```python
from build123d import *

# Parameters (mm, degrees)
BOSS_EXTRUDE1_DEPTH   = 2
BOSS_EXTRUDE2_DEPTH   = 8
SKETCH3_W             = 1.099637712
SKETCH3_H             = 0.808368405
BOSS_EXTRUDE3_DEPTH   = 6
SKETCH4_W             = 1.099637712
SKETCH4_H             = 0.808368405
BOSS_EXTRUDE4_DEPTH   = 6
SKETCH5_W             = 1.099637712
SKETCH5_H             = 0.808368405
BOSS_EXTRUDE5_DEPTH   = 6
SKETCH6_W             = 1.099637712
SKETCH6_H             = 0.808368405
BOSS_EXTRUDE6_DEPTH   = 6
SKETCH7_W             = 4.9
SKETCH7_H             = 6.4
BOSS_EXTRUDE7_DEPTH   = 5
F_1_CLEARANCE_HOLE1_D = 2.20000068
CHAMFER1_SIZE         = 0.2
CHAMFER2_SIZE         = 0.8
FILLET1_R             = 0.8


# Read off the part's stored shape, not the designer's step: Cut-Extrude1, Cut-Extrude2
with BuildPart() as part:
    # Sketch1 → Boss-Extrude1 (new body)
    with BuildSketch(Plane(origin=(0, 0, -2), x_dir=(-1, 0, 0), z_dir=(0, 0, -1))):
        with BuildLine():
            Line((-1.910632622, 9.092570703), (-9.810632622, 9.092570703))
            Line((-9.810632622, 9.092570703), (-9.810632622, 1.192570703))
            ThreePointArc((-9.810632622, 1.192570703), (-11.910632622, -0.907429297), (-9.810632622, -3.007429297))
            Line((-9.810632622, -3.007429297), (-9.810632622, -10.907429297))
            Line((-9.810632622, -10.907429297), (-1.910632622, -10.907429297))
            ThreePointArc((-1.910632622, -10.907429297), (0.189367378, -13.007429297), (2.289367378, -10.907429297))
            Line((2.289367378, -10.907429297), (10.189367378, -10.907429297))
            Line((10.189367378, -10.907429297), (10.189367378, -3.007429297))
            ThreePointArc((10.189367378, -3.007429297), (12.289367378, -0.907429297), (10.189367378, 1.192570703))
            Line((10.189367378, 1.192570703), (10.189367378, 9.092570703))
            Line((10.189367378, 9.092570703), (2.289367378, 9.092570703))
            ThreePointArc((2.289367378, 9.092570703), (0.189367378, 11.192570703), (-1.910632622, 9.092570703))
        make_face()
    extrude(amount=-BOSS_EXTRUDE1_DEPTH)

    # Sketch2 → Boss-Extrude2 (add)
    with BuildSketch(Plane.XY):
        Polygon((-2.670547611, -4.020890836), (-2.670547611, -6.129443348), (-8.453284272, -6.129443348), (-8.453284272, 4.602710154), (-2.670547611, 4.602710154), (-2.670547611, 2.494157643), (-3.670547611, 2.494157643), (-3.670547611, 3.602710154), (-7.453284272, 3.602710154), (-7.453284272, -5.129443348), (-3.670547611, -5.129443348), (-3.670547611, -4.020890836), align=None)
    extrude(amount=BOSS_EXTRUDE2_DEPTH)

    # Sketch3 → Boss-Extrude3 (add)
    with BuildSketch(Plane.XY):
        with Locations((-5.206678265, -1.71002656)):
            Rectangle(SKETCH3_W, SKETCH3_H)
    extrude(amount=BOSS_EXTRUDE3_DEPTH)

    # Sketch4 → Boss-Extrude4 (add)
    with BuildSketch(Plane.XY):
        with Locations((-5.206678265, 2.28997344)):
            Rectangle(SKETCH4_W, SKETCH4_H)
    extrude(amount=BOSS_EXTRUDE4_DEPTH)

    # Sketch5 → Boss-Extrude5 (add)
    with BuildSketch(Plane.XY):
        with Locations((-5.206678265, 0.289973441)):
            Rectangle(SKETCH5_W, SKETCH5_H)
    extrude(amount=BOSS_EXTRUDE5_DEPTH)

    # Sketch6 → Boss-Extrude6 (add)
    with BuildSketch(Plane.XY):
        with Locations((-5.206678265, -3.71002656)):
            Rectangle(SKETCH6_W, SKETCH6_H)
    extrude(amount=BOSS_EXTRUDE6_DEPTH)

    # Sketch7 → Boss-Extrude7 (add)
    with BuildSketch(Plane(origin=(0, 0, -2), x_dir=(-1, 0, 0), z_dir=(0, 0, -1))):
        with Locations((-5.779682622, -0.907429297)):
            Rectangle(SKETCH7_W, SKETCH7_H)
    extrude(amount=BOSS_EXTRUDE7_DEPTH)

    # Cut-Extrude1 outline → Cut-Extrude1 (revolve, cut)
    with BuildSketch(Plane(origin=(5.83567735, -2.101434569, 0), x_dir=(1, 0, 0), z_dir=(0, -1, 0))):
        with BuildLine():
            Line((0.75, -7), (0.75, -6))
            ThreePointArc((0.75, -6), (0.530330086, -6.530330086), (0, -6.75))
            Line((0, -6.75), (0, -7))
            Line((0, -7), (0.75, -7))
        make_face()
    revolve(axis=Axis((5.83567735, -2.101434569, 0), (0, 0, 1)), mode=Mode.SUBTRACT)

    # Cut-Extrude2 outline → Cut-Extrude2 (revolve, cut)
    with BuildSketch(Plane(origin=(5.83567735, 0.898565431, 0), x_dir=(1, 0, 0), z_dir=(0, -1, 0))):
        with BuildLine():
            Line((0.75, -7), (0.75, -6))
            ThreePointArc((0.75, -6), (0.530330086, -6.530330086), (0, -6.75))
            Line((0, -6.75), (0, -7))
            Line((0, -7), (0.75, -7))
        make_face()
    revolve(axis=Axis((5.83567735, 0.898565431, 0), (0, 0, 1)), mode=Mode.SUBTRACT)

    # #1 Clearance Hole1 (through all)
    with Locations(Plane(origin=(0, 0, -2), x_dir=(-1, 0, 0), z_dir=(0, 0, -1))):
        with Locations((0.189367378, -10.907429297), (0.189367378, 9.092570703), (10.189367378, -0.907429297), (-9.810632622, -0.907429297)):
            Hole(F_1_CLEARANCE_HOLE1_D / 2)

    # Chamfer1
    chamfer1_edges = [part.edges().sort_by_distance(p)[0] for p in [
        (-5.206678265, -0.114210762, 6),
        (-4.656859409, 0.28997344, 6),
        (-5.206678265, 0.694157643, 6),
        (-5.756497121, 0.28997344, 6),
        (-5.206678265, -3.305842357, 6),
        (-5.756497121, -3.71002656, 6),
        (-5.206678265, -4.114210762, 6),
        (-4.656859409, -3.71002656, 6),
        (-2.670547611, -4.020890836, 4),
        (-3.670547611, -4.020890836, 4),
        (-3.670547611, 2.494157643, 4),
        (-2.670547611, 2.494157643, 4),
        (-3.170547611, -4.020890836, 8),
        (-3.670547611, -4.575167092, 8),
        (-5.561915941, -5.129443348, 8),
        (-7.453284272, -0.763366597, 8),
        (-5.561915941, 3.602710154, 8),
        (-3.670547611, 3.048433899, 8),
        (-3.170547611, 2.494157643, 8),
        (-2.670547611, 3.548433899, 8),
        (-5.561915941, 4.602710154, 8),
        (-8.453284272, -0.763366597, 8),
        (-5.561915941, -6.129443348, 8),
        (-2.670547611, -5.075167092, 8),
        (-4.656859409, -1.71002656, 6),
        (-5.206678265, -1.305842357, 6),
        (-5.756497121, -1.71002656, 6),
        (-5.206678265, -2.114210762, 6),
        (-4.656859409, 2.28997344, 6),
        (-5.206678265, 2.694157643, 6),
        (-5.756497121, 2.28997344, 6),
        (-5.206678265, 1.885789238, 6),
    ]]
    chamfer(chamfer1_edges, length=CHAMFER1_SIZE)

    # Chamfer2
    chamfer2_edges = [part.edges().sort_by_distance(p)[0] for p in [
        (8.229682622, 2.292570703, -4.5),
    ]]
    chamfer(chamfer2_edges, length=CHAMFER2_SIZE)

    # Fillet1
    fillet1_edges = [part.edges().sort_by_distance(p)[0] for p in [
        (-10.189367378, 9.092570703, -1),
        (-10.189367378, -10.907429297, -1),
        (9.810632622, -10.907429297, -1),
        (9.810632622, 9.092570703, -1),
    ]]
    fillet(fillet1_edges, radius=FILLET1_R)


solid = part.part
```
Part model, mm, in its own coordinate system. A direction names the side the tool comes from. Coordinates: 2 decimals unless noted, no trailing zeros. Order: outer loops, then holes, each group sorted by start corner. A loop starts at its lowest first (then second) coordinate and runs counter-clockwise, first axis right, second up. Notation, with made-up numbers: (75.25, -24.5) -> (126.25, -24.5) arc R24 cw to (126.25, -9.5) -> close; hole circle Ø7 at (58.5, 67.5). An arc over 180 degrees is marked (long way). Put each result on its own line as item: value. Start each with the question number.
(1) Mould opens along X. For faces 1 (the face through (-4.657, 0.3, 2.9)), 2 (the face through (6, -1, -7)), 3 (the face through (-5.756, 0.3, 2.9)), 4 (the face through (-6, 3.603, 4)) say: pulls with the +X half, pulls with the -X half, needs draft (parallel to the pull), parting line crosses it, or undercut.
(2) Band-saw the part on A-A (z = 4.5). Count the separate pieces of the cut face and the enclosed holes in it, then the cut area to 3 significant figures.
(3) Band-saw the part on C-C (z = -3). Give the cut face in (x, y).
(4) Which spindle directions (+Z, -Z, +X, -X, +Y, -Y) get a long thin tool onto all of the face, cutting with end or side? Do faces 5 (the face through (-6, -6.129, 4)), 6 (the face through (-6, 9.093, -1)), 7 (the face through (-5, 2.694, 3)), 8 (the face through (-5, -2.114, 3)). Say none if no direction does.
(5) Probe line 1 along X through (y, z) = (3.5, 1.25); line 2 along X through (y, z) = (0.5, 2.75); line 3 along X through (y, z) = (4, 3.25). List the from-to ranges inside material, lowest first. Write a range as [from, to].
(6) Band-saw the part on B-B (x = -4). Give the cut face in (y, z), then the cut area to 3 significant figures.
(7) Band-saw the part on D-D (y = -9.5). Give the cut face in (x, z), then the cut area to 3 significant figures.
(8) Pin check, flat tips, straight feed: pin 1 Ø2 at (y, z) = (6.5, -0.5) entering from +X; pin 2 Ø0.9 at (x, z) = (-5.5, 2.5) entering from -Y; pin 3 Ø1.2 at (x, z) = (-5, 4) entering from +Y; pin 4 Ø1.8 at (x, y) = (-0.19, -10.91) entering from -Z. Stop position of each tip, or through.
Determined:
1. face 1: pulls with the +X half
1. face 2: needs draft
1. face 3: undercut
1. face 4: undercut
2. separate pieces: 5
2. enclosed holes: 0
2. area: 26.0 mm²
3. outline: (3.33, -4.11) -> (8.23, -4.11) -> (8.23, 1.49) -> (7.43, 2.29) -> (3.33, 2.29) -> close
4. face 5: +Z, +X, -X, -Y
4. face 6: +Z, -Z, -X, +Y
4. face 7: +Z
4. face 8: +Z, +X
5. line 1: x = [-8.45, -7.45], [-3.67, -2.67]
5. line 2: x = [-8.45, -7.45], [-5.76, -4.66]
5. line 3: x = [-8.45, -2.67]
6. outline: (-10.91, -2) -> (9.09, -2) -> (9.09, 0) -> (4.6, 0) -> (4.6, 7.8) -> (4.4, 8) -> (3.8, 8) -> (3.6, 7.8) -> (3.6, 0) -> (-5.13, 0) -> (-5.13, 7.8) -> (-5.33, 8) -> (-5.93, 8) -> (-6.13, 7.8) -> (-6.13, 0) -> (-10.91, 0) -> close
6. area: 55.9 mm²
7. outline: (-10.19, -2) -> (9.81, -2) -> (9.81, 0) -> (-10.19, 0) -> close
7. area: 40.0 mm²
8. pin 1: stops at x = 9.81
8. pin 2: stops at y = -6.13
8. pin 3: stops at y = 4.6
8. pin 4: passes through
